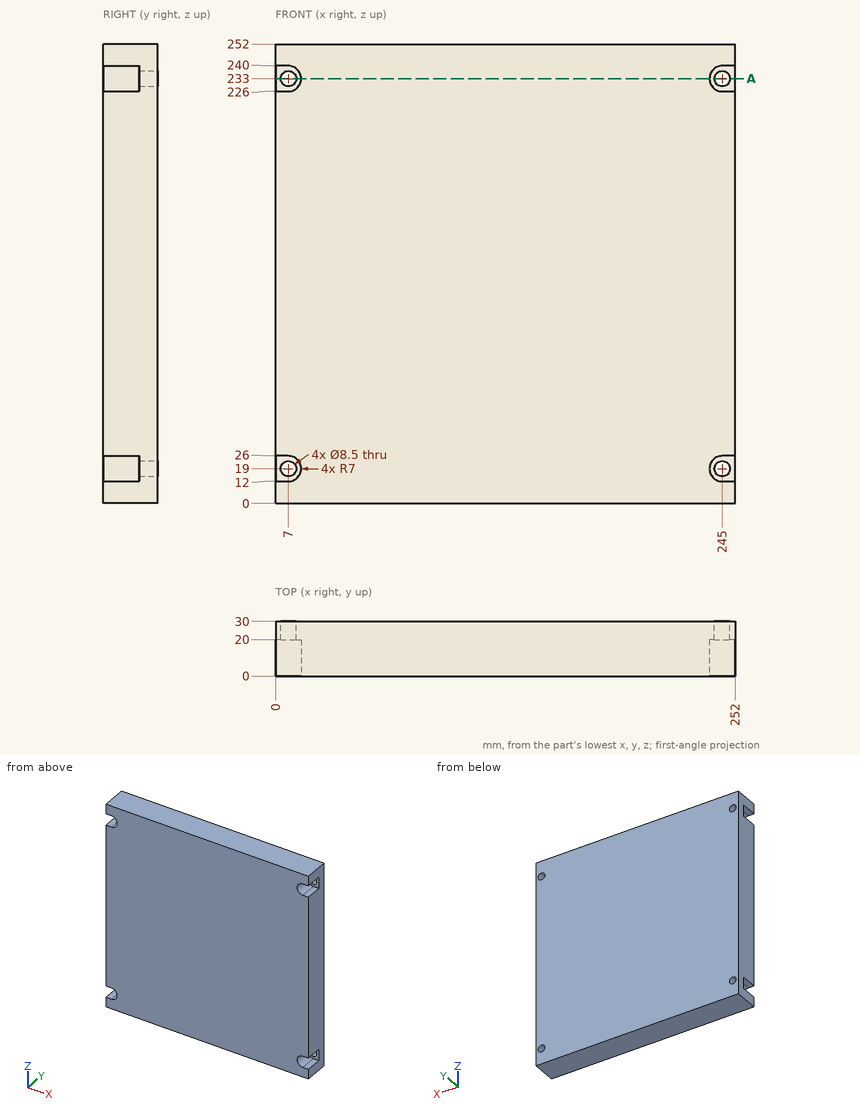
Geometry check sheet. Reference: drawing and pictorial views, mm from the part's lowest x, y, z. Coordinates: 2 decimals unless noted, no trailing zeros. Loops run counter-clockwise (first coordinate to the right, second up) from the corner with the lowest first, then second, coordinate; pieces in that order, holes last. Notation, with made-up numbers: (58.5, 28.25) - (103.5, 28.25) arc R9 cw to (103.5, 36.25) - close; hole circle Ø9 at (66, -6). An arc over 180 degrees is marked (long way). Return JSON: item names as keys, results as strings.
1. Thickness scan on L1, parallel to Z at x = 7, y = 25.5. Record the ranges inside material, lowest first.
Established:
{"L1": "z = 0 to 14.75, 23.25 to 228.75, 237.25 to 252"}
2. Section check A-A, the plane z = 233. Record the boundary of the cut face in (x, y), then the cut area to 3 significant figures.
Established:
{"outline": "(0, 20) - (2.75, 20) - (2.75, 30) - (0, 30) - close; (11.25, 20) - (14, 20) - (14, 0) - (238, 0) - (238, 20) - (240.75, 20) - (240.75, 30) - (11.25, 30) - close; (249.25, 20) - (252, 20) - (252, 30) - (249.25, 30) - close", "area": "6,830 mm2"}
3. Go/stop test with flat-tipped pins: pin 1 (7.5 mm diameter, centred on x = 7, z = 233, fed in from -Y); pin 2 (11 mm diameter, centred on x = 4, z = 18.5, fed in from -Y). Record where each tip stops, or that it passes through.
Established:
{"pin 1": "passes through", "pin 2": "stops at y = 20"}
